Verification items for this drawing (mm, ordinates from the low corner). Give positions to 0.01 mm unless a question says otherwise; leave off trailing zeros. Loops run counter-clockwise (first coordinate to the right, second up) from the corner with the lowest first, then second, coordinate; pieces in that order, holes last. Notation, with made-up numbers: M 27.5,1 L 39.5,1 A14 ccw 39.5,24 Z; hole C 87.25,-31 d11. An arc over 180 degrees is marked long. Answer in a Markdown table with one row per item.
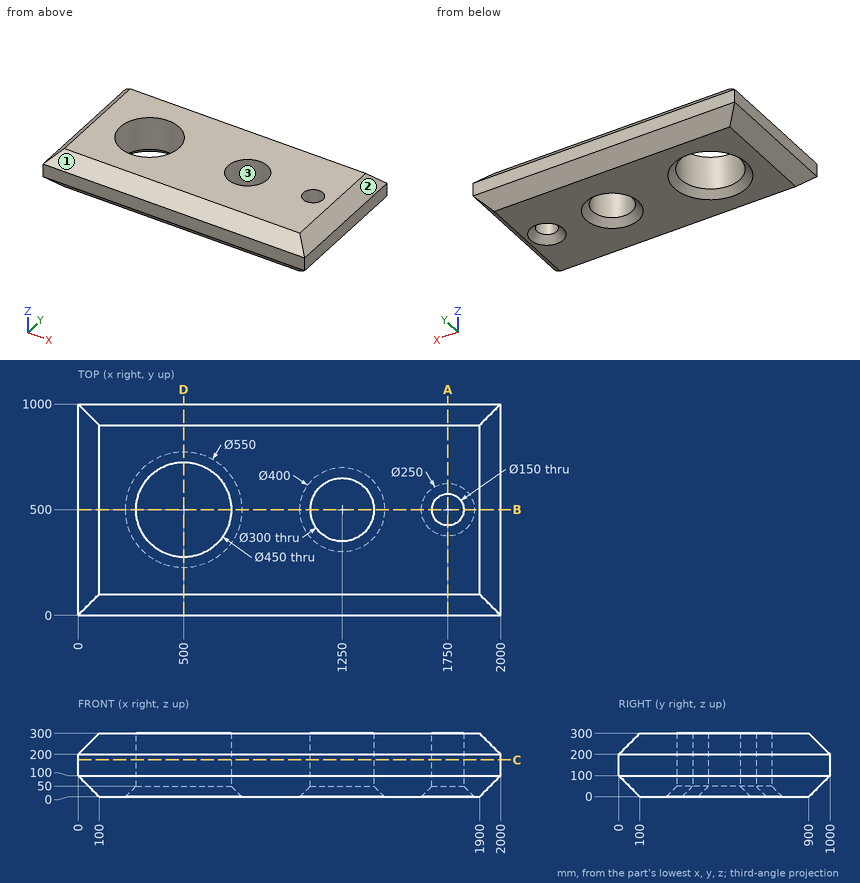
Item 1: Scan lines: L1, parallel to X at y = 367.5, z = 81; L2, parallel to Y at x = 500, z = 142.5; L3, parallel to Y at x = 1250, z = 183. Record each from-to range of solid material in increasing order. Write a range as [from, to].
Reported:
| item | result |
|---|---|
| L1 | x = [19, 318.15], [681.85, 1179.69], [1320.31, 1981] |
| L2 | y = [0, 275], [725, 1000] |
| L3 | y = [0, 350], [650, 1000] |
Item 2: Go/stop test with flat-tipped pins: pin 1 (10 mm diameter, centred on y = 443, z = 56, fed in from +X); pin 2 (8 mm diameter, centred on y = 599.5, z = 47, fed in from -X); pin 3 (12 mm diameter, centred on y = 792, z = 30.5, fed in from -X). Record where each tip stops, or that it passes through.
Reported:
| item | result |
|---|---|
| pin 1 | stops at x = 1961 |
| pin 2 | stops at x = 49 |
| pin 3 | stops at x = 63.5 |
Item 3: Sectioned sample at B-B (y = 500). Record the cut outline in (x, z).
Reported:
| item | result |
|---|---|
| outline | M 0,100 L 100,0 L 225,0 L 275,50 L 275,300 L 100,300 L 0,200 Z; M 725,50 L 775,0 L 1050,0 L 1100,50 L 1100,300 L 725,300 Z; M 1400,50 L 1450,0 L 1625,0 L 1675,50 L 1675,300 L 1400,300 Z; M 1825,50 L 1875,0 L 1900,0 L 2000,100 L 2000,200 L 1900,300 L 1825,300 Z |
Item 4: Sectioned sample at C-C (z = 174). Record the cut outline in (x, y), and give its area (3 significant figures).
Reported:
| item | result |
|---|---|
| outline | M 0,0 L 2000,0 L 2000,1000 L 0,1000 Z; hole C 500,500 d450; hole C 1250,500 d300; hole C 1750,500 d150 |
| area | 1,750,000 mm^2 |
Item 5: Sectioned sample at D-D (x = 500). Record the cut outline in (y, z).
Reported:
| item | result |
|---|---|
| outline | M 0,100 L 100,0 L 225,0 L 275,50 L 275,300 L 100,300 L 0,200 Z; M 725,50 L 775,0 L 900,0 L 1000,100 L 1000,200 L 900,300 L 725,300 Z |
Item 6: Sectioned sample at A-A (x = 1750). Record the cut outline in (y, z).
Reported:
| item | result |
|---|---|
| outline | M 0,100 L 100,0 L 375,0 L 425,50 L 425,300 L 100,300 L 0,200 Z; M 575,50 L 625,0 L 900,0 L 1000,100 L 1000,200 L 900,300 L 575,300 Z |
Item 7: Release check for a two-part mould opening along X. For the marked faces 1, 2 and 3 record: released by +X, released by -X, zero draft, split by the parting line, or undercut.
Reported:
| item | result |
|---|---|
| face 1 | zero draft |
| face 2 | released by +X |
| face 3 | undercut |
